Solid Edge part; units mm, degrees
sketch "Sketch1" plane through (0, 0, 0) normal (0, -1, 0) x (1, 0, 0)
  line L0 (-25, -12.5) -> (25, -12.5)
  arc A0 (25, 12.5) -> (25, -12.5) centre (25, 0) cw
  line L1 (25, 12.5) -> (-25, 12.5)
  arc A1 (-25, 12.5) -> (-25, -12.5) centre (-25, 0) ccw
  dimension "D1" = 25
extrude "Protrusion1" add sketch "Sketch1" against normal blind 3
sketch "Sketch2" plane through (0, 0, 0) normal (0, -1, 0) x (1, 0, 0)
  circle A0 centre (-25, 0) radius 11
  circle A1 centre (25, 0) radius 11
extrude "Extrusionsausprägung_2" add sketch "Sketch2" against normal blind 15
sketch "Sketch3" plane through (0, 3, 0) normal (0, 1, 0) x (1, 0, 0)
  circle A0 centre (0, 0) radius 11
extrude "Extrusionsausprägung_3" add sketch "Sketch3" along normal blind 20
properties material "Polykarbonat"
Verification items for the finished model (mm, model axes). A direction names the side the tool comes from. Give positions to 0.01 mm unless a question says otherwise; leave off trailing zeros. Order: outer loops, then holes, each group sorted by start corner. A loop starts at its lowest first (then second) coordinate and runs counter-clockwise, first axis right, second up. Notation, with made-up numbers: M 2.25,-7.75 L 26.25,-7.75 A17 cw 26.25,-3.75 Z; hole C -16,20 d5. An arc over 180 degrees is marked long. Return JSON: item names as keys, results as strings. Group by question number.
1) Access from +Z, -Z, +X, -X, +Y, -Y to the whole of each face (thin tool, end or side, straight path). Record for faces 1 (the face through (35.161, 8.916, -4.213)), 2 (the face through (25, 15, 0)), 3 (the face through (0, 1, -12.5)).
2) Go/stop test with flat-tipped pins: pin 1 Ø2 at (y, z) = (8.5, -3.5) entering from -X; pin 2 Ø4 at (x, y) = (-22, 11) entering from +Z; pin 3 Ø12 at (y, z) = (5.5, -10) entering from +X. Record where each tip stops, or that it passes through.
3) Section check D-D on y = 20.5. Record the cut outline in (x, z), and give its area (3 significant figures).
4) Scan lines: line 1 (X direction, y = 10.5, z = -1); line 2 (X direction, y = 3.75, z = -7.5); line 3 (Y direction, x = -18.5, z = 4.25). Record each from-to range of solid material in increasing order.
5) Mould release check, pull along X, two halves, no side actions. Record for faces 4 (the face through (-37.497, 1.479, 0.275)), 5 (the face through (-2.38, 12.86, -10.74)), 6 (the face through (-25, 15, 0)): pulls with the +X half, pulls with the -X half, needs draft (parallel to the pull), parting line crosses it, or undercut.
6) Section check C-C on x = 0. Record the cut outline in (y, z), and give its area (3 significant figures).
7) Section check A-A on z = 0. Record the cut outline in (x, y).
8) Section check B-B on y = 9.75. Record the cut outline in (x, z), and give its area (3 significant figures).
Answer block:
{
 "1": {"face 1": "+Y", "face 2": "+Z, -Z, +X, +Y", "face 3": "-Z, +X, -X, +Y, -Y"},
 "2": {"pin 1": "stops at x = -35.71", "pin 2": "stops at z = 10.95", "pin 3": "stops at x = 36.64"},
 "3": {"outline": "C 0,0 d22", "area": "380 mm^2"},
 "4": {"line 1": "x = -35.95 to -14.05, -10.95 to 10.95, 14.05 to 35.95", "line 2": "x = -33.05 to -16.95, -8.05 to 8.05, 16.95 to 33.05", "line 3": "y = 0 to 15"},
 "5": {"face 4": "pulls with the -X half", "face 5": "undercut", "face 6": "needs draft"},
 "6": {"outline": "M 0,-12.5 L 3,-12.5 L 3,-11 L 23,-11 L 23,11 L 3,11 L 3,12.5 L 0,12.5 Z", "area": "515 mm^2"},
 "7": {"outline": "M -37.5,0 L 37.5,0 L 37.5,3 L 36,3 L 36,15 L 14,15 L 14,3 L 11,3 L 11,23 L -11,23 L -11,3 L -14,3 L -14,15 L -36,15 L -36,3 L -37.5,3 Z"},
 "8": {"outline": "C -25,0 d22; C 0,0 d22; C 25,0 d22", "area": "1,140 mm^2"}
}
